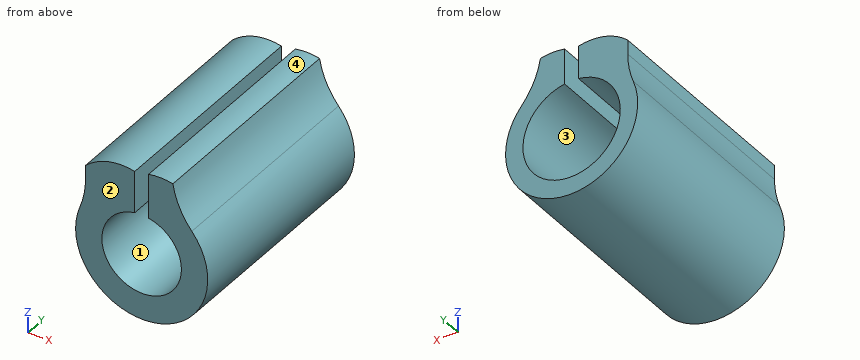
```python
from build123d import *

# Parameters (mm, degrees)
BOSS_EXTRUDE1_DEPTH = 78
SKETCH2_R           = 17.5
CUT_EXTRUDE1_DEPTH  = 39
FILLET1_R           = 30


with BuildPart() as part:
    # Sketch1 → Boss-Extrude1 (new body)
    with BuildSketch(Plane(origin=(0, 0, 0), x_dir=(1, 0, 0), z_dir=(0, 1, 0))):
        with BuildLine():
            Line((2.5, -14.079772725), (2.5, -21.006468516))
            Line((2.5, -21.006468516), (2.5, -30.076468516))
            ThreePointArc((2.5, -30.076468516), (6.86, -30.550052571), (11.22, -30.076468516))
            Line((11.22, -30.076468516), (11.22, -20.932608533))
            ThreePointArc((11.22, -20.932608533), (6.153268827, 22.93904494), (-20.19, -12.50705401))
            Line((-20.19, -12.50705401), (-20.19, -24.339979577))
            ThreePointArc((-20.19, -24.339979577), (-11.948714524, -28.965226171), (-2.5, -29.148218549))
            Line((-2.5, -29.148218549), (-2.5, -21.006468516))
            Line((-2.5, -21.006468516), (-2.5, -14.079772725))
            ThreePointArc((-2.5, -14.079772725), (0, 14.3), (2.5, -14.079772725))
        make_face()
    extrude(amount=BOSS_EXTRUDE1_DEPTH)

    # Sketch2 → Cut-Extrude1 (cut)
    with BuildSketch(Plane(origin=(0, 78, 0), x_dir=(1, 0, 0), z_dir=(0, 1, 0))):
        Circle(SKETCH2_R)
    extrude(amount=-CUT_EXTRUDE1_DEPTH, mode=Mode.SUBTRACT)

    # Fillet1
    # the kernel refuses this fillet: 30 mm, written as the material it adds along each edge
    with BuildSketch(Plane(origin=(11.22, 0, 20.932608533), x_dir=(0.7793190463800559, 0, -0.626627340569561), z_dir=(0, 1, 0))) as fillet1_piece_1:
        with BuildLine():
            CenterArc((14.269740905, -29.487081198), FILLET1_R, 100.610162443, 31.198957304)
            Line((-5.729792663, -7.125984242), (-6.129783335, -6.678762303))
            ThreePointArc((-6.129783335, -6.678762303), (-3.33248776, -3.187015717), (-0.467591428, 0.375976404))
            Line((-0.467591428, 0.375976404), (0.110475413, 0.589741624))
            ThreePointArc((0.110475413, 0.589741624), (4.372985116, 0.193939281), (8.635494818, 0.589741624))
            Line((8.635494818, 0.589741624), (8.745970232, 0))
        make_face()
    extrude(amount=78)
    with BuildSketch(Plane(origin=(-20.19, 0, 12.50705401), x_dir=(0, 0, 1), z_dir=(0, 1, 0))) as fillet1_piece_2:
        with BuildLine():
            CenterArc((6.729016275, -30), FILLET1_R, 90, 20.970079677)
            Line((-4.007395047, -1.986976744), (-4.222123273, -1.426716279))
            ThreePointArc((-4.222123273, -1.426716279), (-2.22334858, -0.55048945), (-0.31596768, 0.510063158))
            Line((-0.31596768, 0.510063158), (0, 0.6))
            Line((0, 0.6), (6.729016275, 0.6))
            Line((6.729016275, 0.6), (6.729016275, 0))
        make_face()
    extrude(amount=78)


solid = part.part
```
Part model, mm, in its own coordinate system. Face numbers are marked on the shaded views. Coordinates: 2 decimals unless noted, no trailing zeros. Loops run counter-clockwise (first coordinate to the right, second up) from the corner with the lowest first, then second, coordinate; pieces in that order, holes last. Notation, with made-up numbers: (70.5, 89.5) - (129.5, 89.5) arc R12 ccw to (129.5, 95.5) - close; hole circle Ø9 at (27, 6.5). An arc over 180 degrees is marked (long way). Write item = value, one per line. Start each with the question number.
Item 1: Cut at B-B, the plane x = -7.5. Give the cut face in (y, z).
Item 2: Cut at C-C, the plane y = 11.5. Give the cut face in (x, z).
Item 3: Cut at D-D, the plane x = 0. Give the cut face in (y, z), and give its area (3 significant figures).
Item 4: Wall check: L1, parallel to X at y = 63, z = 0; L2, parallel to X at y = 22, z = 0; L3, parallel to Y at x = 10, z = -12.5. Give the ranges that are in metal, low to high. Write a range as from..to.
Item 5: Cut at A-A, the plane z = 0. Give the cut face in (x, y), and give its area (3 significant figures).
Item 6: Mould opens along Z. For the marked faces 1, 2, 3 and 4 say: released by +Z, released by -Z, zero draft, split by the parting line, or undercut.
Item 7: Flat gauge pins, fed straight in: pin 1 Ø2.5 at (y, z) = (40, 22.5) entering from -X; pin 2 Ø1 at (x, y) = (4.5, 58.5) entering from -Z; pin 3 Ø5 at (y, z) = (34, 8) entering from +X. Where does each tip first touch, or does it go through?
The answers:
q1.outline = (0, -22.53) - (78, -22.53) - (78, -15.81) - (39, -15.81) - (39, -12.18) - (0, -12.18) - close; (0, 12.18) - (39, 12.18) - (39, 15.81) - (78, 15.81) - (78, 29.63) - (0, 29.63) - close
q2.outline = (-22.18, 8.5) arc R23.75 ccw (long way) to (18.04, 15.45) arc R30 cw to (11.22, 30.08) arc R20.31 ccw to (2.5, 30.08) - (2.5, 14.08) arc R14.3 cw (long way) to (-2.5, 14.08) - (-2.5, 29.15) arc R19.4 ccw to (-20.19, 24.34) - (-20.19, 19.24) arc R30 cw to start
q3.outline = (0, -23.75) - (78, -23.75) - (78, -17.5) - (39, -17.5) - (39, -14.3) - (0, -14.3) - close
q3.area = 612 mm2
q4.L1 = -23.75..-17.5, 17.5..23.75
q4.L2 = -23.75..-14.3, 14.3..23.75
q4.L3 = 0..39
q5.outline = (-23.75, 0) - (-14.3, 0) - (-14.3, 39) - (-17.5, 39) - (-17.5, 78) - (-23.75, 78) - close; (14.3, 0) - (23.75, 0) - (23.75, 78) - (17.5, 78) - (17.5, 39) - (14.3, 39) - close
q5.area = 1,220 mm2
q6.face_1 = undercut
q6.face_2 = zero draft
q6.face_3 = undercut
q6.face_4 = released by +Z
q7.pin_1 = -20.19
q7.pin_2 = -23.41
q7.pin_3 = 23.1
